Check sheet for the modelled part. Datum: model origin and axes. Units: mm. A direction names the side the tool comes from. Round coordinates to 2 decimals unless told otherwise and drop trailing zeros. Write each loop counter-clockwise with the first axis right and the second up, starting at its lowest first coordinate (ties: lowest second). Pieces come first, ordered by that corner, then holes. Notation, with made-up numbers: M -27,38.5 L 30,38.5 A20 ccw 30,47.5 Z; hole C -19.75,-34 d3. An arc over 180 degrees is marked long. Answer in a Markdown table with one row per item.
Autodesk Inventor part; units mm, degrees
ref_plane "YZ Plane" through (0, 0, 0) normal (1, 0, 0) x (0, 1, 0)
ref_plane "XZ Plane" through (0, 0, 0) normal (0, 1, 0) x (-1, 0, 0)
ref_plane "XY Plane" through (0, 0, 0) normal (0, 0, 1) x (1, 0, 0)
sketch "Sketch1" plane through (0, 0, 0) normal (0, 0, 1) x (1, 0, 0)
  circle A0 centre (0, 0) radius 2.6
  dimension "d0" = 5.2
extrude "Extrusion1" add sketch "Sketch1" along normal blind 1
sketch "Sketch2" plane through (0, 0, 1) normal (0, 0, 1) x (1, 0, 0)
  circle A0 centre (0, 0) radius 2
  dimension "d3" = 4
extrude "Extrusion2" add sketch "Sketch2" along normal blind 4
thread "Thread1"
chamfer "Chamfer2" distance 0.5 angle 45 1 edges at (-2.6, 0, 1)
properties part number "M4x5flat"
1. Section check A-A, the plane y = 0. Record the cut outline in (x, z), and give its area (4 significant figures).
Found:
| item | result |
|---|---|
| outline | M -2.6,0 L 2.6,0 L 2.6,0.5 L 2.1,1 L 2,1 L 2,5 L -2,5 L -2,1 L -2.1,1 L -2.6,0.5 Z |
| area | 20.95 mm2 |
2. Section check C-C, the plane z = 0.85. Record the cut outline in (x, y).
Found:
| item | result |
|---|---|
| outline | C 0,0 d4.5 |
3. Scan lines: L1, parallel to X at y = 0.05, z = 2.55; L2, parallel to X at y = 1.7, z = 2.9; L3, parallel to Z at x = -1.8, y = 1.8. Record each from-to range of solid material in increasing order.
Found:
| item | result |
|---|---|
| L1 | x = -2 to 2 |
| L2 | x = -1.05 to 1.05 |
| L3 | z = 0 to 0.55 |
4. Section check D-D, the plane z = 4.7. Record the cut outline in (x, y), and give its area (3 significant figures).
Found:
| item | result |
|---|---|
| outline | C 0,0 d4 |
| area | 12.6 mm2 |
5. Access from +Z, -Z, +X, -X, +Y, -Y to the whole of each face (thin tool, end or side, straight path). Record for faces 1 (the face through (0, 2, 3)), 2 (the face through (0, 0, 0)).
Found:
| item | result |
|---|---|
| face 1 | +Z |
| face 2 | -Z, +X, -X, +Y, -Y |
